Autodesk Inventor part; units mm, degrees
ref_plane "YZ Plane" through (0, 0, 0) normal (1, 0, 0) x (0, 1, 0)
ref_plane "XZ Plane" through (0, 0, 0) normal (0, 1, 0) x (-1, 0, 0)
ref_plane "XY Plane" through (0, 0, 0) normal (0, 0, 1) x (1, 0, 0)
sketch "スケッチ1" plane through (0, 0, 0) normal (1, 0, 0) x (0, 1, 0)
  line L0 (125.6523, 179.1954) -> (-64.3477, 179.1954)
  line L1 (-64.3477, 179.1954) -> (-64.3477, -110.8046)
  line L2 (-64.3477, -110.8046) -> (125.6523, -110.8046)
  line L3 (125.6523, -110.8046) -> (125.6523, 179.1954)
  point P0 (0, 0)
  dimension "d0" = 190
  dimension "d1" = 290
extrude "押し出し1" add sketch "スケッチ1" along normal blind 2.6
sketch "スケッチ2" plane through (2.6, 0, 0) normal (1, 0, 0) x (0, 0, -1)
  line L0 (-179.1954, 125.6523) -> (-179.1954, -64.3477)
  line L1 (-179.1954, -64.3477) -> (110.8046, -64.3477)
  line L2 (110.8046, -64.3477) -> (110.8046, 125.6523)
  line L3 (110.8046, 125.6523) -> (-179.1954, 125.6523)
  line L4 (-34.1954, 30.6523) -> (-34.1954, 125.6523)
  line L5 (110.8046, 125.6523) -> (-179.1954, 125.6523)
  line L6 (-34.1954, 30.6523) -> (110.8046, 30.6523)
  point P0 (0, 0)
  point P1 (-169.1954, 115.6523)
  point P2 (100.8046, 115.6523)
  point P3 (-169.1954, -54.3477)
  point P4 (100.8046, -54.3477)
  dimension "d4" = 10
  dimension "d5" = 10
hole "穴1" at (2.6, 115.6523, 169.1954) at (2.6, 115.6523, -100.8046) at (2.6, -54.3477, 169.1954) at (2.6, -54.3477, -100.8046) direction (-1, 0, 0) diameter 4.5 depth 10 tip angle 118
sketch "スケッチ6" plane through (0, 0, 0) normal (-1, 0, 0) x (0, 0, 1)
  circle A0 centre (129.1954, -14.3477) radius 29.75
  circle A1 centre (129.1954, 65.6523) radius 25
  line L0 (-80.8046, -19.4977) -> (85.9954, -19.4977)
  line L1 (85.9954, -19.4977) -> (85.9954, 80.8023)
  line L2 (85.9954, 80.8023) -> (-80.8046, 80.8023)
  line L3 (-80.8046, 80.8023) -> (-80.8046, -19.4977)
  point P0 (0, 0)
extrude "押し出し5" cut sketch "スケッチ6" against normal up to surface (2.6 mm away)
properties part number "lc_box_side" material "ポリカーボネート、クリア"
The model under review builds one solid part; all positions refer to its coordinate system, in mm. Round coordinates to 2 decimals unless told otherwise and drop trailing zeros. Write each loop counter-clockwise with the first axis right and the second up, starting at its lowest first coordinate (ties: lowest second). Pieces come first, ordered by that corner, then holes. Notation, with made-up numbers: (35.25, 17) - (68.25, 17) arc R19 cw to (68.25, 26) - close; hole circle Ø3 at (-23.75, -2). An arc over 180 degrees is marked (long way). One line per item, written item: value. Start each with the question number.
1. Consider section B-B on y = 27.5. Write out the cut boundary in (x, z), and give its area (3 significant figures).
2. Consider section D-D on y = 58.5. Write out the cut boundary in (x, z).
3. To check wall thickness, follow L1, parallel to Z at x = 0.3, y = -13; L2, parallel to Z at x = 1.1, y = -11; L3, parallel to Y at x = 0.1, z = -17. State the ranges of each line that lie inside material, in increasing order. Write a range as from..to.
4. Consider section C-C on x = 0.85. Write out the cut boundary in (y, z), and give its area (3 significant figures).
5. Consider section A-A on z = 71. Write out the cut boundary in (x, y), and give its area (3 significant figures).
Checks:
1. outline: (0, -110.8) - (2.6, -110.8) - (2.6, -80.8) - (0, -80.8) - close; (0, 86) - (2.6, 86) - (2.6, 179.2) - (0, 179.2) - close
1. area: 320 mm^2
2. outline: (0, -110.8) - (2.6, -110.8) - (2.6, -80.8) - (0, -80.8) - close; (0, 86) - (2.6, 86) - (2.6, 105.24) - (0, 105.24) - close; (0, 153.15) - (2.6, 153.15) - (2.6, 179.2) - (0, 179.2) - close
3. L1: z = -110.8..-80.8, 86..99.48, 158.91..179.2
3. L2: z = -110.8..-80.8, 86..99.63, 158.76..179.2
3. L3: y = -64.35..-19.5, 80.8..125.65
4. outline: (-64.35, -110.8) - (125.65, -110.8) - (125.65, 179.2) - (-64.35, 179.2) - close; hole circle Ø4.5 at (-54.35, -100.8); hole circle Ø4.5 at (-54.35, 169.2); hole circle Ø59.5 at (-14.35, 129.2); hole (-19.5, -80.8) - (80.8, -80.8) - (80.8, 86) - (-19.5, 86) - close; hole circle Ø50 at (65.65, 129.2); hole circle Ø4.5 at (115.65, -100.8); hole circle Ø4.5 at (115.65, 169.2)
4. area: 33,600 mm^2
5. outline: (0, -64.35) - (2.6, -64.35) - (2.6, -19.5) - (0, -19.5) - close; (0, 80.8) - (2.6, 80.8) - (2.6, 125.65) - (0, 125.65) - close
5. area: 233 mm^2
